The figure shows three views and two pictorial views of one solid part (mm, origin at its lowest corner). Answer the questions. A direction names the side the tool comes from. Give positions to 0.01 mm unless a question says otherwise; leave off trailing zeros. Loops run counter-clockwise (first coordinate to the right, second up) from the corner with the lowest first, then second, coordinate; pieces in that order, holes last. Notation, with made-up numbers: M -26,-36.5 L -3,-36.5 A9 ccw -3,-24.5 Z; hole C -7,34 d11. An arc over 180 degrees is marked long. One line per item, written item: value. Start each with the question number.
Q1. A cutting plane is placed at C-C, the plane z = 2.5. Determine the outline of the cut face in (x, y), and give its area (3 significant figures).
Q2. The mould has two halves that part along Y. Classify the marked faces 3, 4 and 5: +Y half, -Y half, draft (parallel to the pull), parting line (faces both ways), or undercut.
Q3. Flat-ended cylindrical pins translate along their axes: pin 1 (2 mm diameter, centred on x = 25, z = 4, fed in from +Y); pin 2 (1 mm diameter, centred on x = 23, z = 8, fed in from -Y). Find the tip coordinate at first contact, or state that the pin passes through.
Q4. For the marked faces 1 and 2, determine the directions among +Z, -Z, +X, -X, +Y, -Y from which every point of the face is accessible in a straight line to the end or side of a thin tool.
Q5. Consider L1, parallel to Y at x = 17.25, z = 6.75; L2, parallel to Y at x = 13, z = 5.25. Determine where each line is inside the solid, lowest interval first.
Q6. A cutting plane is placed at A-A, the plane y = 17.25. Determine the outline of the cut face in (x, z).
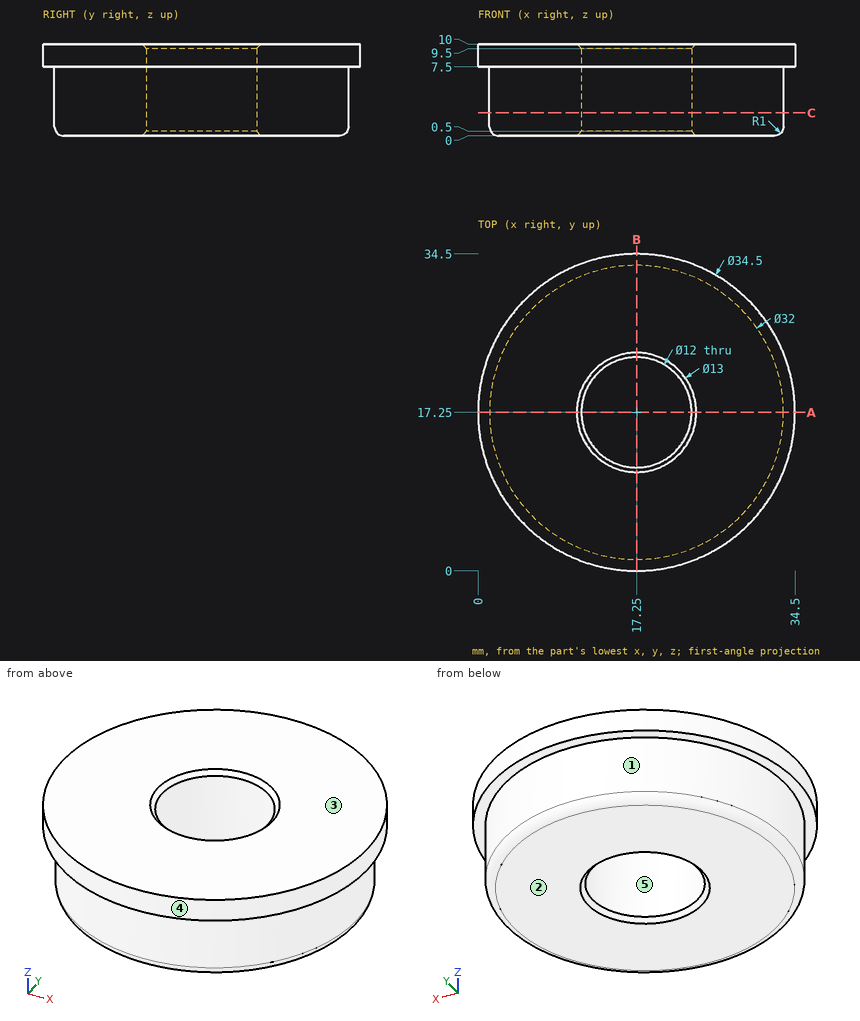
Answer block:
1. outline: C 17.25,17.25 d32; hole C 17.25,17.25 d12
1. area: 691 mm^2
2. face 3: draft
2. face 4: parting line
2. face 5: undercut
3. pin 1: y = 31.76
3. pin 2: y = 0.82
4. face 1: -Z
4. face 2: -Z, +X, -X, +Y, -Y
5. L1: 1.25 to 11.25, 23.25 to 33.25
5. L2: 1.82 to 13.01, 21.49 to 32.68
6. outline: M 0,7.5 L 1.25,7.5 L 1.25,1 A1 ccw 2.25,0 L 10.75,0 L 11.25,0.5 L 11.25,9.5 L 10.75,10 L 0,10 Z; M 23.25,0.5 L 23.75,0 L 32.25,0 A1 ccw 33.25,1 L 33.25,7.5 L 34.5,7.5 L 34.5,10 L 23.75,10 L 23.25,9.5 Z
